Work out the finished part from the listing and answer in its coordinate system (mm). Coordinates: 2 decimals unless noted, no trailing zeros. Loops run counter-clockwise (first coordinate to the right, second up) from the corner with the lowest first, then second, coordinate; pieces in that order, holes last. Notation, with made-up numbers: (14.5, -11) -> (63.5, -11) arc R23 ccw to (63.5, 18) -> close; hole circle Ø9 at (43, -15). An arc over 180 degrees is marked (long way). Use a Markdown table: item, result. Add a question column.
```python
from build123d import *

# Parameters (mm, degrees)
F0_W     = 10
F0_H     = 141.806
F1_DEPTH = 495
F3_DEPTH = 10
F5_DEPTH = 10


with BuildPart() as f1:
    # F0 (on Top) → F1 (new body)
    with BuildSketch(Plane.XY):
        with Locations((-37.828005, 12.564924)):
            Rectangle(F0_W, F0_H)
    extrude(amount=F1_DEPTH)

    # F2 (on face) → F3 (cut)
    with BuildSketch(Plane(origin=(-42.828005, 0, 0), x_dir=(0, -1, 0), z_dir=(-1, 0, 0))):
        Polygon((-83.467924, 0), (48.338076, 0), (-83.467924, 495), align=None)
        Polygon((-74.296774, 495), (58.338076, 0), (58.338076, 495), align=None)
    extrude(amount=-F3_DEPTH, mode=Mode.SUBTRACT)

    # F4 (on face) → F5 (join)
    with BuildSketch(Plane(origin=(-42.828005, 0, 0), x_dir=(0, -1, 0), z_dir=(-1, 0, 0))):
        Polygon((-83.467924, 505), (-83.467924, 495), (-74.296774, 495), align=None)
    extrude(amount=-F5_DEPTH)


solid = f1.part
```
Item 1: Section A-A (x = -35.75) is taken. Determine the outline of the cut face in (y, z), then the cut area to 3 significant figures.
Item 2: Section C-C (y = 56.5) is taken. Determine the outline of the cut face in (x, z), then the cut area to 3 significant figures.
Item 3: Given pin 1 (1.5 mm diameter, centred on x = -41.5, z = 196, fed in from +Y); pin 2 (4 mm diameter, centred on x = -39, z = 180.5, fed in from +Y); pin 3 (1.5 mm diameter, centred on x = -36, z = 63.5, fed in from -Y), each flat-ended and moving along its own axis, determine where each tip first touches the part or whether it passes through.
Item 4: Section B-B (z = 277) is taken. Determine the outline of the cut face in (x, y).
Item 5: Find the intervals of material crossed by probe 1 along Y at (x, z) = (-36.5, 107); probe 2 along Y at (x, z) = (-38.75, 327.5), in increasing order.
Output:
| question | item | result |
|---|---|---|
| 1 | outline | (-58.34, 0) -> (-48.34, 0) -> (83.47, 495) -> (83.47, 505) -> (74.3, 495) -> close |
| 1 | area | 4,790 mm2 |
| 2 | outline | (-42.83, 393.72) -> (-32.83, 393.72) -> (-32.83, 428.58) -> (-42.83, 428.58) -> close |
| 2 | area | 349 mm2 |
| 3 | pin 1 | stops at y = 4.05 |
| 3 | pin 2 | stops at y = 0.26 |
| 3 | pin 3 | stops at y = -41.52 |
| 4 | outline | (-42.83, 15.88) -> (-32.83, 15.88) -> (-32.83, 25.42) -> (-42.83, 25.42) -> close |
| 5 | probe 1 | y = -29.67 to -19.85 |
| 5 | probe 2 | y = 29.42 to 38.87 |
